Source: CAD feature listing. Evaluate the final solid. Frame: model axes, mm. A direction names the side the tool comes from. Round coordinates to 2 decimals unless told otherwise and drop trailing zeros. Loops run counter-clockwise (first coordinate to the right, second up) from the corner with the lowest first, then second, coordinate; pieces in that order, holes last. Notation, with made-up numbers: M -12.5,32.25 L 40.5,32.25 A21 cw 40.5,65.25 Z; hole C 45,-3 d2. An arc over 180 degrees is marked long. Answer as CSV lines item,"result". Start each with the question number.
```python
from build123d import *

# Parameters (mm, degrees)
IZIM2_R                     = 48.5
IZIM2_R_2                   = 1.5
Y_KSEKLIK_EKSTR_ZYON1_DEPTH = 4
Y_KSEKLIK_EKSTR_ZYON2_DEPTH = 20
KES_EKSTR_ZYON2_DEPTH       = 9
KES_EKSTR_ZYON4_DEPTH       = 18
IZIM8_R                     = 8.999373408
KES_EKSTR_ZYON6_DEPTH       = 20
IZIM10_R                    = 1.3
KES_EKSTR_ZYON7_DEPTH       = 13
Y_KSEKLIK_EKSTR_ZYON3_DEPTH = 12
RADYUS1_R                   = 3
RADYUS2_R                   = 3
IZIM11_W                    = 10
IZIM11_H                    = 4
KES_EKSTR_ZYON8_DEPTH       = 6
IZIM12_R                    = 4.00063253
KES_EKSTR_ZYON9_DEPTH       = 2
KES_EKSTR_ZYON10_DEPTH      = 40
KES_EKSTR_ZYON10_DEPTH_BACK = 40


with BuildPart() as part:
    # Çizim2 → Yükseklik-Ekstrüzyon1 (new body)
    with BuildSketch(Plane(origin=(0, 0, 0), x_dir=(1, 0, 0), z_dir=(0, 1, 0))):
        with Locations(Location((0, -4, 0), (0, 0, 270))):
            Circle(IZIM2_R)
        with Locations(Location((7.25, -4, 0), (0, 0, 270))):
            Circle(IZIM2_R_2, mode=Mode.SUBTRACT)
        with Locations(Location((-7.25, -4, 0), (0, 0, 270))):
            Circle(IZIM2_R_2, mode=Mode.SUBTRACT)
    extrude(amount=-Y_KSEKLIK_EKSTR_ZYON1_DEPTH)

    # Çizim3 → Yükseklik-Ekstrüzyon2 (add)
    with BuildSketch(Plane.XY):
        with BuildLine():
            Line((31.238930549, 26.071347433), (3.495879159, 53.755241116))
            ThreePointArc((3.495879159, 53.755241116), (-32.936073069, 51.72385839), (-26.943926702, 15.730694583))
            ThreePointArc((-26.943926702, 15.730694583), (-21.379626349, 8.847295043), (-21.118861947, 0))
            Line((-21.118861947, 0), (-8.860527496, 0))
            Line((-8.860527496, 0), (38.580138623, 0))
            Line((38.580138623, 0), (38.580138623, 8.374820438))
            ThreePointArc((38.580138623, 8.374820438), (36.672018128, 17.954230697), (31.238930549, 26.071347433))
        make_face()
    extrude(amount=-Y_KSEKLIK_EKSTR_ZYON2_DEPTH)

    # Çizim5 → Kes-Ekstrüzyon2 (cut)
    with BuildSketch(Plane(origin=(0, 0, -20), x_dir=(-1, 0, 0), z_dir=(0, 0, -1))):
        with BuildLine():
            Line((-29.580138623, 0), (-29.580138623, 8.355768388))
            ThreePointArc((-29.580138623, 8.355768388), (-29.424047841, 10.115726146), (-28.960648361, 11.820741267))
            ThreePointArc((-28.960648361, 11.820741267), (-23.965436041, 23.095860189), (-17.588526551, 33.651213249))
            ThreePointArc((-17.588526551, 33.651213249), (-17.177321901, 34.202292772), (-16.7292201, 34.72381236))
            Line((-16.7292201, 34.72381236), (0, 52.891150841))
            ThreePointArc((0, 52.891150841), (32.164197471, 47.609241385), (22.142551812, 16.593103896))
            ThreePointArc((22.142551812, 16.593103896), (14.125970591, 9.960582753), (11.118861947, 0))
            Line((11.118861947, 0), (-29.580138623, 0))
        make_face()
    extrude(amount=-KES_EKSTR_ZYON2_DEPTH, mode=Mode.SUBTRACT)

    # Çizim7 → Kes-Ekstrüzyon4 (cut)
    with BuildSketch(Plane(origin=(0, 0, -20), x_dir=(-1, 0, 0), z_dir=(0, 0, -1))):
        Polygon((28.483058649, 36.490937082), (0, 7), (-15.105114115, 21.588883698), (13.377944534, 51.079820781), align=None)
    extrude(amount=-KES_EKSTR_ZYON4_DEPTH, mode=Mode.SUBTRACT)

    # Çizim8 → Kes-Ekstrüzyon6 (cut)
    with BuildSketch(Plane(origin=(0, 0, -20), x_dir=(-1, 0, 0), z_dir=(0, 0, -1))):
        with Locations((13.809736929, 36.412644661)):
            Circle(IZIM8_R)
    extrude(amount=-KES_EKSTR_ZYON6_DEPTH, mode=Mode.SUBTRACT)

    # Çizim10 → Kes-Ekstrüzyon7 (cut)
    with BuildSketch(Plane(origin=(0, 0, -20), x_dir=(-1, 0, 0), z_dir=(0, 0, -1))):
        with Locations((-13.580138623, 15.2501239)):
            Circle(IZIM10_R)
        with Locations((-6.318582157, 8.374820438)):
            Circle(IZIM10_R)
        with Locations((19.765881259, 49.77609902)):
            Circle(IZIM10_R)
        with Locations((27.027437725, 42.900795558)):
            Circle(IZIM10_R)
    extrude(amount=-KES_EKSTR_ZYON7_DEPTH, mode=Mode.SUBTRACT)

    # 3B Çizim1 → Yükseklik-Ekstrüzyon3 (add)
    with BuildSketch(Plane(origin=(29.714278279, 0, 2), x_dir=(-0.35112344158839165, 0, 0.9363291775690447), z_dir=(0, 1, 0))):
        Polygon((0, 0), (14.981266841, 5.617975065), (17.088007491, 0), (2.10674065, -5.617975065), align=None)
    extrude(amount=Y_KSEKLIK_EKSTR_ZYON3_DEPTH)

    # Radyus1
    radyus1_edges = [part.edges().sort_by_distance(p)[0] for p in [
        (26.714278279, 12, 18),
    ]]
    fillet(radyus1_edges, radius=RADYUS1_R)

    # Radyus2
    radyus2_edges = [part.edges().sort_by_distance(p)[0] for p in [
        (26.714278279, 12, 2),
    ]]
    fillet(radyus2_edges, radius=RADYUS2_R)

    # Çizim11 → Kes-Ekstrüzyon8 (cut)
    with BuildSketch(Plane(origin=(29.714278279, 0, 0), x_dir=(0, 0, -1), z_dir=(1, 0, 0))):
        with Locations((-9.980022365, 6)):
            Rectangle(IZIM11_W, IZIM11_H)
    extrude(amount=-KES_EKSTR_ZYON8_DEPTH, mode=Mode.SUBTRACT)

    # Çizim12 → Kes-Ekstrüzyon9 (cut)
    with BuildSketch(Plane(origin=(0, -4, 0), x_dir=(-1, 0, 0), z_dir=(0, -1, 0))):
        with Locations(Location((0.071138185, -4, 0), (0, 0, 90))):
            Circle(IZIM12_R)
    extrude(amount=-KES_EKSTR_ZYON9_DEPTH, mode=Mode.SUBTRACT)

    # Çizim13 → Kes-Ekstrüzyon10 (cut, two sides)
    with BuildSketch(Plane(origin=(0, 0, 0), x_dir=(0, 0, -1), z_dir=(1, 0, 0))) as kes_ekstr_zyon10_sk:
        with BuildLine():
            Line((16, 60.912644661), (25.8774704, 60.912644661))
            Line((25.8774704, 60.912644661), (25.8774704, 0))
            Line((25.8774704, 0), (20, 0))
            add(Edge.make_bspline(
                [(16, 60.912644661), (16.195964828, 30.341679785), (20, 0)],
                knots=[0, 0, 0, 1, 1, 1], degree=2))
        make_face()
    extrude(amount=KES_EKSTR_ZYON10_DEPTH, mode=Mode.SUBTRACT)
    extrude(kes_ekstr_zyon10_sk.sketch, amount=-KES_EKSTR_ZYON10_DEPTH_BACK, mode=Mode.SUBTRACT)


solid = part.part
```
1) Access query for faces 4 (the flat face through (38.58, 4, -10)), 5 (the flat face through (27, 4, 18)), 6 (the cylindrical face through (1.131, -3.014, 0.184)). Directions: +Z, -Z, +X, -X, +Y, -Y. A direction counts if a zero-diameter tool reaches every point of the face in a straight line with its end or side. Return the directions, or none.
2) Section B-B, the plane z = -25. Return loops of the section in (x, y).
3) Contact query for flat-ended pins moving along their axis: pin 1 Ø7 at (x, z) = (-0.07, 4) entering from -Y; pin 2 Ø5 at (x, z) = (26.5, 11) entering from +Y; pin 3 Ø13 at (y, z) = (7, 10) entering from -X; pin 4 Ø9 at (x, z) = (-1.5, 5) entering from -Y. Output: stop coordinate, or through.
4) Section A-A, the plane x = -7.25. Give the number of separate pieces and of enclosed holes in the cut face, and give its area (3 significant figures).
5) Ray query, line 1 along X through (y, z) = (-3, 4); line 2 along Z through (x, y) = (3, 37); line 3 along Y through (x, z) = (14, -17.5). Return the intervals inside material, ascending.
6) Mould query, pull axis Z, two halves, no side actions, for faces 1 (the flat face through (-20, 50, -7)), 2 (the cylindrical face through (-8.58, -1.97, 4.69)), 3 (the cylindrical face through (-4.82, 36.81, -1.01)). Classes: pulls with the +Z half, pulls with the -Z half, needs draft (parallel to the pull), parting line crosses it, or undercut.
Findings below:
1,face 4,"+Z, -Z, +X, +Y"
1,face 5,"+Z, +X, -X, +Y"
1,face 6,"-Y"
2,outline,"M -38.87,-4 L 38.87,-4 L 38.87,0 L -38.87,0 Z"
3,pin 1,"y = -2"
3,pin 2,"y = 12"
3,pin 3,"x = 23.71"
3,pin 4,"y = -4"
4,separate pieces,"3"
4,enclosed holes,"0"
4,area,"751 mm²"
5,line 1,"-48.5 to -8.75, -5.75 to -4.07, 3.93 to 5.75, 8.75 to 48.5"
5,line 2,"-11 to 0"
5,line 3,"-4 to 0"
6,face 1,"pulls with the -Z half"
6,face 2,"undercut"
6,face 3,"needs draft"
